```python
from build123d import *

# Parameters (mm, degrees)
SKETCH2_R          = 5.3
CUT_EXTRUDE1_START = -5.75
CUT_EXTRUDE1_DEPTH = 4.5
CUT_EXTRUDE2_START = -7
SKETCH6_R          = 5.475
SKETCH6_R_2        = 3.5
CUT_EXTRUDE2_DEPTH = 20
CHAMFER1_SIZE      = 1
CHAMFER2_SIZE      = 0.5


with BuildPart() as part:
    # Sweep1: sweep along a path in Sketch1
    with BuildLine(Plane.XY) as sweep1_path:
        Line((0, 0), (0, 64.5))
        ThreePointArc((0, 64.5), (17.5, 82), (35, 64.5))
        Line((35, 64.5), (35, 27.5))
    # Sketch2 → Sweep1 (sweep)
    with BuildSketch(Plane(origin=(0, 0, 0), x_dir=(1, 0, 0), z_dir=(0, 1, 0))):
        Circle(SKETCH2_R)
    sweep(path=sweep1_path.line)

    # Sketch4 → Cut-Extrude1 (cut)
    with BuildSketch(Plane.XZ.offset(-27.5).offset(CUT_EXTRUDE1_START)):
        with BuildLine():
            Line((29.815407441, 1.1), (40.184592559, 1.1))
            ThreePointArc((40.184592559, 1.1), (35, 5.3), (29.815407441, 1.1))
        make_face()
    extrude(amount=-CUT_EXTRUDE1_DEPTH, mode=Mode.SUBTRACT)

    # Sketch6 → Cut-Extrude2 (cut)
    with BuildSketch(Plane.XZ.offset(CUT_EXTRUDE2_START)):
        Circle(SKETCH6_R)
        with Locations(Location((0, 0, 0), (0, 0, 270))):
            Circle(SKETCH6_R_2, mode=Mode.SUBTRACT)
    extrude(amount=-CUT_EXTRUDE2_DEPTH, mode=Mode.SUBTRACT)

    # Chamfer1
    chamfer1_edges = [part.edges().sort_by_distance(p)[0] for p in [
        (40.3, 27.5, 0),
        (-5.3, 7, 0),
        (-5.3, 27, 0),
        (-5.3, 0, 0),
    ]]
    chamfer(chamfer1_edges, length=CHAMFER1_SIZE)

    # Chamfer2
    chamfer2_edges = [part.edges().sort_by_distance(p)[0] for p in [
        (35, 37.75, 5.3),
        (35, 33.25, 5.3),
    ]]
    chamfer(chamfer2_edges, length=CHAMFER2_SIZE)


solid = part.part
```
Read the model definition and answer for the solid it produces. Units are mm, in the model's axes. A direction names the side the tool comes from. Coordinates: 2 decimals unless noted, no trailing zeros. Loops run counter-clockwise (first coordinate to the right, second up) from the corner with the lowest first, then second, coordinate; pieces in that order, holes last. Notation, with made-up numbers: (66, 23) - (98, 23) arc R21 cw to (98, 43) - close; hole circle Ø10 at (-31, -27). An arc over 180 degrees is marked (long way). Answer in a Markdown table with one row per item.
1. Given pin 1 (1.1 mm diameter, centred on x = 36, z = 3, fed in from -Y); pin 2 (4 mm diameter, centred on x = 37, z = 3, fed in from +Y); pin 3 (4 mm diameter, centred on x = 18, z = -4, fed in from -Y), each flat-ended and moving along its own axis, determine where each tip first touches the part or whether it passes through.
Conclusion:
| item | result |
|---|---|
| pin 1 | stops at y = 27.5 |
| pin 2 | stops at y = 78.16 |
| pin 3 | stops at y = 77.08 |
2. Find section A-A, the plane y = 56. Write down the section's boundary in (x, z), then the cut area to 3 significant figures.
Conclusion:
| item | result |
|---|---|
| outline | circle Ø10.6 at (0, 0); circle Ø10.6 at (35, 0) |
| area | 176 mm² |
3. Which of the six approach directions +Z, -Z, +X, -X, +Y, -Y give full straight-line access (tool end or side, diameter ignored) to faces 5 (the face through (35.094, 37.885, 4.934)), 6 (the face through (0, 0, 0)), 7 (the face through (4.896, 3.535, 2.03)), 8 (the face through (35, 37.75, 3))?
Conclusion:
| item | result |
|---|---|
| face 5 | +Z |
| face 6 | +Z, -Z, +X, -X, -Y |
| face 7 | -Y |
| face 8 | +Z, +X |
4. Determine the mould class of faces 1 (the face through (35, 27.5, 0)), 2 (the face through (35.094, 33.115, 4.934)), 3 (the face through (35.69, 46.248, -5.255)), 4 (the face through (-3.417, 16.86, 0.759)) for opening direction X: +X half, -X half, draft (parallel to the pull), parting line (faces both ways), or undercut.
Conclusion:
| item | result |
|---|---|
| face 1 | draft |
| face 2 | undercut |
| face 3 | undercut |
| face 4 | parting line |
5. Find section C-C, the plane y = 22.5. Write down the section's boundary in (x, z).
Conclusion:
| item | result |
|---|---|
| outline | circle Ø7 at (0, 0) |
6. Straight lines are drawn through the part: line 1 (X direction, y = 34.5, z = 0.25); line 2 (X direction, y = 28, z = -3.25); line 3 (X direction, y = 11.5, z = 0). For each, find the intervals that lie inside material, in ascending order.
Conclusion:
| item | result |
|---|---|
| line 1 | x = -5.29 to 5.29, 29.71 to 40.29 |
| line 2 | x = -4.19 to 4.19, 31.47 to 38.53 |
| line 3 | x = -3.5 to 3.5 |
7. Find section B-B, the plane z = 0. Write down the section's boundary in (x, y), then the cut area to 3 significant figures.
Conclusion:
| item | result |
|---|---|
| outline | (-5.3, 1) - (-4.3, 0) - (4.3, 0) - (5.3, 1) - (5.3, 6) - (4.3, 7) - (3.5, 7) - (3.5, 27) - (4.3, 27) - (5.3, 28) - (5.3, 64.5) arc R12.2 cw to (29.7, 64.5) - (29.7, 28.5) - (30.7, 27.5) - (39.3, 27.5) - (40.3, 28.5) - (40.3, 64.5) arc R22.8 ccw to (-5.3, 64.5) - (-5.3, 28) - (-4.3, 27) - (-3.5, 27) - (-3.5, 7) - (-4.3, 7) - (-5.3, 6) - close |
| area | 1,580 mm² |
